from build123d import *

# Parameters (mm, degrees)
ESQUISSE3_W             = 9.75
ESQUISSE3_H             = 2.4
ENL_V_MAT_EXTRU_1_DEPTH = 5
BOSS_EXTRU_1_START      = -12
ESQUISSE2_R             = 1.25
BOSS_EXTRU_1_DEPTH      = 10
ENL_V_MAT_EXTRU_2_DEPTH = 5


with BuildPart() as part:
    # Esquisse1 → Révolution1 (revolve)
    with BuildSketch(Plane.XY, mode=Mode.PRIVATE) as r_volution1_sk:
        with BuildLine():
            Line((-2.5, 0), (-3.75, 0))
            ThreePointArc((-3.75, 0), (-2.025351028, 3.15601857), (1.562241714, 3.409090909))
            ThreePointArc((1.562241714, 3.409090909), (3.596212455, 2.729915791), (5.728219619, 2.5))
            Line((5.728219619, 2.5), (14.25, 2.5))
            Line((14.25, 2.5), (14.25, 1.25))
            Line((14.25, 1.25), (4.5, 1.25))
            Line((4.5, 1.25), (4.5, 0))
            Line((4.5, 0), (2.5, 0))
            ThreePointArc((2.5, 0), (0, 2.5), (-2.5, 0))
        make_face()
    revolve(r_volution1_sk.sketch.rotate(Axis((4.5, 0, 0), (1, 0, 0)), 90), axis=Axis((4.5, 0, 0), (1, 0, 0)))

    # Esquisse3 → Enlèv. mat.-Extru.1 (cut, symmetric)
    with BuildSketch(Plane.XY):
        with Locations((1.125, 2.8)):
            Rectangle(ESQUISSE3_W, ESQUISSE3_H)
        with Locations((1.125, -2.8)):
            Rectangle(ESQUISSE3_W, ESQUISSE3_H)
    extrude(amount=ENL_V_MAT_EXTRU_1_DEPTH, both=True, mode=Mode.SUBTRACT)

    # Esquisse2 → Boss.-Extru.1 (add)
    with BuildSketch(Plane(origin=(14.25, 0, 0), x_dir=(0, 0, -1), z_dir=(1, 0, 0)).offset(BOSS_EXTRU_1_START)):
        Polygon((0, 2.886751346), (-2.5, 1.443375673), (-2.5, -1.443375673), (0, -2.886751346), (2.5, -1.443375673), (2.5, 1.443375673), align=None)
        with Locations(Location((0, 0, 0), (0, 0, 180))):
            Circle(ESQUISSE2_R, mode=Mode.SUBTRACT)
    extrude(amount=BOSS_EXTRU_1_DEPTH)

    # Esquisse4 → Enlèv. mat.-Extru.2 (cut, symmetric)
    with BuildSketch(Plane.XY):
        Polygon((2.771281292, 1.6), (5, 2.886751346), (-3.75, 2.886751346), (-3.75, 1.6), align=None)
        Polygon((-3.75, -1.6), (2.771281292, -1.6), (5, -2.886751346), (-3.75, -2.886751346), align=None)
    extrude(amount=ENL_V_MAT_EXTRU_2_DEPTH, both=True, mode=Mode.SUBTRACT)


solid = part.part
CAD build for the part. Positions are in the model's coordinates, mm. A direction names the side the tool comes from. Round coordinates to 2 decimals unless told otherwise and drop trailing zeros. Order: outer loops, then holes, each group sorted by start corner. A loop starts at its lowest first (then second) coordinate and runs counter-clockwise, first axis right, second up. Notation, with made-up numbers: (-20, -26) -> (28, -26) arc R31 cw to (28, 4) -> close; hole circle Ø4 at (66, 82). An arc over 180 degrees is marked (long way). Write each question's results on one line, items separated by ' | '.
1. Cut at A-A (x = -0.25). Give the cut face in (y, z), plus the area to 3 significant figures.
Findings below:
outline: (-1.6, -3.38) arc R3.74 ccw to (1.6, -3.38) -> (1.6, -1.9) arc R2.49 cw to (-1.6, -1.9) -> close; (-1.6, 1.9) arc R2.49 cw to (1.6, 1.9) -> (1.6, 3.38) arc R3.74 ccw to (-1.6, 3.38) -> close | area: 8.45 mm²
2. Pull direction Y, two halves, no side cores. Call faces 1 (the face through (13.3, -0.1, -2.5)), 2 (the face through (9.31, -0.05, -1.25)), 3 (the face through (8.497, -2.175, -1.233)): pulls with the +Y half, pulls with the -Y half, needs draft (parallel to the pull), parting line crosses it, or undercut.
Findings below:
face 1: parting line crosses it | face 2: undercut | face 3: pulls with the -Y half
3. 3-axis set-ups, long thin cutter, end or side, ignore diameter. For faces 4 (the face through (7.444, 2.155, -1.268)), 5 (the face through (14.25, -1, 1)), 6 (the face through (7.444, -2.155, 1.268)), 7 (the face through (4.5, 0, 0)), 8 (the face through (12.25, 1.328, 2.295)): which of +Z, -Z, +X, -X, +Y, -Y reach the whole face in a straight line?
Findings below:
face 4: -Z, +X, +Y | face 5: +Z, -Z, +X, +Y, -Y | face 6: +Z, +X, -Y | face 7: +X | face 8: +Z, +X, +Y
4. Flat gauge pins, fed straight in: P1, Ø1.2, axis at y = 0.5, z = -0.5, coming from the +X side; P2, Ø1.5, axis at x = -0.5, z = 2.5, coming from the +Y side; P3, Ø2, axis at y = 1, z = 0.5, coming from the -X side; P4, Ø3, axis at x = 7, y = -0.5, coming from the +Z side. Where does each tip first touch, or does it go through?
Findings below:
P1: stops at x = 14.25 | P2: stops at y = 1.6 | P3: stops at x = -3.75 | P4: stops at z = 2.5
5. Cut at D-D (x = 5.25). Give the cut face in (y, z), plus the area to 3 significant figures.
Findings below:
outline: (-2.89, 0) -> (-1.44, -2.5) -> (-0.24, -2.5) arc R2.51 ccw to (0.24, -2.5) -> (1.44, -2.5) -> (2.89, 0) -> (1.44, 2.5) -> (0.24, 2.5) arc R2.51 ccw to (-0.24, 2.5) -> (-1.44, 2.5) -> close; hole circle Ø2.5 at (0, 0) | area: 16.7 mm²
6. Cut at B-B (x = 8.5). Give the cut face in (y, z), plus the area to 3 significant figures.
Findings below:
outline: (-2.89, 0) -> (-1.44, -2.5) -> (1.44, -2.5) -> (2.89, 0) -> (1.44, 2.5) -> (-1.44, 2.5) -> close; hole circle Ø2.5 at (0, 0) | area: 16.7 mm²
7. Wall check: line 1 along Y through (x, z) = (11.75, 0.75); line 2 along Z through (x, y) = (3.25, 1.35); line 3 along Z through (x, y) = (-0.75, 1.2). Give the ranges that are in metal, low to high. Write a range as [from, to].
Findings below:
line 1: y = [-2.45, -1], [1, 2.45] | line 2: z = [-2.5, 2.5] | line 3: z = [-3.47, -2.06], [2.06, 3.47]
